```python
from build123d import *

# Parameters (mm, degrees)
F1_DEPTH = 508
F2_R     = 1.524
F3_R     = 3.9624


with BuildPart() as f1:
    # F0 (on Front) → F1 (new body)
    with BuildSketch(Plane.XZ):
        Polygon((7.950636, 9.393655), (7.950636, 7.488655), (20.320436, 7.488655), (20.320436, -6.786145), (58.445836, -6.786145), (58.445836, 247.213855), (56.540836, 247.213855), (56.540836, -4.881145), (22.225436, -4.881145), (22.225436, 9.393655), align=None)
    extrude(amount=-F1_DEPTH)

    # F2
    f2_edges = [f1.edges().sort_by_distance(p)[0] for p in [
        (20.320436, 254, 7.488655),
        (22.225436, 254, -4.881145),
        (56.540836, 254, -4.881145),
    ]]
    fillet(f2_edges, radius=F2_R)

    # F3
    f3_edges = [f1.edges().sort_by_distance(p)[0] for p in [
        (22.225436, 254, 9.393655),
        (20.320436, 254, -6.786145),
        (58.445836, 254, -6.786145),
    ]]
    fillet(f3_edges, radius=F3_R)


solid = f1.part
```
The model under review builds one solid part; all positions refer to its coordinate system, in mm. A direction names the side the tool comes from. Give positions to 0.01 mm unless a question says otherwise; leave off trailing zeros. Write each loop counter-clockwise with the first axis right and the second up, starting at its lowest first coordinate (ties: lowest second). Pieces come first, ordered by that corner, then holes. Notation, with made-up numbers: (-21, 50.25) - (11, 50.25) arc R27 ccw to (11, 71.25) - close; hole circle Ø8 at (48.25, 38). An arc over 180 degrees is marked (long way). Answer in a Markdown table with one row per item. Add a question column.
1. We need section A-A on y = 392.5. Write out the cut boundary in (x, z), then the cut area to 3 significant figures.
2. Insertion check: P1, Ø9.5, axis at x = 43.5, y = 207, coming from the +Z side; P2, Ø10, axis at y = 100.5, z = 144, coming from the -X side; P3, Ø1, axis at x = 14, y = 298.5, coming from the +Z side. Each pin has a flat end and moves straight along its axis. Give the tip position at first contact, or say it passes through.
3. Draft analysis for pull direction X (two halves, no side actions). For faces 4 (the flat face through (57, 0, 93)), 5 (the flat face through (22.225, 250, 1)), 6 (the flat face through (20.32, 250, 2)), 7 (the flat face through (40, 250, -4.881)), state which applies: +X half, -X half, draft (parallel to the pull), parting line (faces both ways), or undercut.
4. Tool access review of faces 1 (the flat face through (13, 250, 9.394)), 2 (the flat face through (58.446, 250, 120)), 3 (the flat face through (13, 250, 7.489)): name each direction out of +Z, -Z, +X, -X, +Y, -Y from which nothing blocks a thin tool from reaching the whole face with its end or side.
5. Wall thickness on line 1 along Z through (x, y) = (32.5, 319.5); line 2 along X through (y, z) = (236.5, 56); line 3 along Z through (x, y) = (16.5, 216): over which ranges is each line inside the solid? List them lowest first. Write a range as [from, to].
6. We need section B-B on x = 36. Write out the cut boundary in (y, z).
7. We need section C-C on z = 95. Write out the cut boundary in (x, y).
Ans:
| question | item | result |
|---|---|---|
| 1 | outline | (7.95, 7.49) - (18.8, 7.49) arc R1.52 cw to (20.32, 5.96) - (20.32, -2.82) arc R3.96 ccw to (24.28, -6.79) - (54.48, -6.79) arc R3.96 ccw to (58.45, -2.82) - (58.45, 247.21) - (56.54, 247.21) - (56.54, -3.36) arc R1.52 cw to (55.02, -4.88) - (23.75, -4.88) arc R1.52 cw to (22.23, -3.36) - (22.23, 5.43) arc R3.96 ccw to (18.26, 9.39) - (7.95, 9.39) - close |
| 1 | area | 595 mm^2 |
| 2 | P1 | stops at z = -4.88 |
| 2 | P2 | stops at x = 56.54 |
| 2 | P3 | stops at z = 9.39 |
| 3 | face 4 | draft |
| 3 | face 5 | undercut |
| 3 | face 6 | -X half |
| 3 | face 7 | undercut |
| 4 | face 1 | +Z, -X, +Y, -Y |
| 4 | face 2 | +Z, -Z, +X, +Y, -Y |
| 4 | face 3 | -Z, -X, +Y, -Y |
| 5 | line 1 | z = [-6.79, -4.88] |
| 5 | line 2 | x = [56.54, 58.45] |
| 5 | line 3 | z = [7.49, 9.39] |
| 6 | outline | (0, -6.79) - (508, -6.79) - (508, -4.88) - (0, -4.88) - close |
| 7 | outline | (56.54, 0) - (58.45, 0) - (58.45, 508) - (56.54, 508) - close |
